Geometry: final body of the model. Coordinates: model frame, mm. A direction names the side the tool comes from. Round coordinates to 2 decimals unless told otherwise and drop trailing zeros. Loops run counter-clockwise (first coordinate to the right, second up) from the corner with the lowest first, then second, coordinate; pieces in that order, holes last. Notation, with made-up numbers: (-0.75, 48) - (13.25, 48) arc R19 cw to (13.25, 65) - close; hole circle Ø4 at (16.5, 23.5). An arc over 180 degrees is marked (long way). Write item = value, one per line. Start each with the question number.
Item 1: First-contact query: pin 1 (3 mm diameter, centred on x = 12.5, y = -5, fed in from -Z); pin 2 (8 mm diameter, centred on y = -6, z = 22, fed in from +X); pin 3 (1 mm diameter, centred on x = 26, y = 5, fed in from -Z). Flat tips, straight axial feed; report the tip coordinate or a pass-through.
Item 2: Draft query along X for faces 3 (the cylindrical face through (-7.493, 0.33, 31.406)), 4 (the flat face through (50, 0, 0)). Return one class per face: pulls with the +X half, pulls with the -X half, needs draft (parallel to the pull), parting line crosses it, or undercut.
Item 3: Line query: line 1 (X direction, y = 0.5, z = 55); line 2 (X direction, y = 5, z = 37); line 3 (Y direction, x = 43.5, z = 55). Output: solid intervals per line, ascending. Write a range as from..to.
Item 4: Section A-A (z = 36). Return loops of the section in (x, y).
Item 5: Access query for faces 1 (the cylindrical face through (42.846, 2.253, 30.594)), 2 (the flat face through (0, 0, 0)). Directions: +Z, -Z, +X, -X, +Y, -Y. A direction counts if a zero-diameter tool reaches every point of the face in a straight line with its end or side. Return the directions, or none.
Item 6: Section B-B (y = 0). Return loops of the section in (x, z).
from build123d import *

# Parameters (mm, degrees)
F1_R    = 7.5
F3_SIZE = 2


with BuildPart() as f2:
    # F2: sweep along a path in F0
    with BuildLine(Plane.XZ) as f2_path:
        Line((0, 0), (0, 60))
        ThreePointArc((0, 60), (25, 85), (50, 60))
        Line((50, 60), (50, 0))
    # F1 (on Top) → F2 (sweep)
    with BuildSketch(Plane.XY):
        Circle(F1_R)
    sweep(path=f2_path.line)

    # F3
    f3_edges = [f2.edges().sort_by_distance(p)[0] for p in [
        (-7.5, 0, 0),
        (57.5, 0, 0),
    ]]
    chamfer(f3_edges, length=F3_SIZE)


solid = f2.part
Taken from the geometry:
q1.pin_1 = 72.75
q1.pin_2 = 57.23
q1.pin_3 = 78.97
q2.face_3 = undercut
q2.face_4 = needs draft
q3.line_1 = -7.48..7.48, 42.52..57.48
q3.line_2 = -5.59..5.59, 44.41..55.59
q3.line_3 = -3.74..3.74
q4.outline = circle Ø15 at (0, 0); circle Ø15 at (50, 0)
q5.face_1 = -Z
q5.face_2 = -Z, +X, -X, +Y, -Y
q6.outline = (-7.5, 2) - (-5.5, 0) - (5.5, 0) - (7.5, 2) - (7.5, 60) arc R17.5 cw to (42.5, 60) - (42.5, 2) - (44.5, 0) - (55.5, 0) - (57.5, 2) - (57.5, 60) arc R32.5 ccw to (-7.5, 60) - close
